Geometry: final body of the model. Coordinates: model frame, mm. Face numbers are marked on the shaded views. A direction names the side the tool comes from. Coordinates: 2 decimals unless noted, no trailing zeros. Loops run counter-clockwise (first coordinate to the right, second up) from the corner with the lowest first, then second, coordinate; pieces in that order, holes last. Notation, with made-up numbers: (27.25, -29.75) - (62.25, -29.75) arc R17 cw to (62.25, -9.75) - close; hole circle Ø8 at (42, -14.75). An arc over 180 degrees is marked (long way). Answer in a Markdown table with one row per item.
from build123d import *

# Parameters (mm, degrees)
F0_R     = 60
F1_DEPTH = 30


with BuildPart() as f1:
    # F0 (on Front) → F1 (new body)
    with BuildSketch(Plane.XZ):
        with BuildLine():
            Line((-23.376703, 94.018714), (-93.376703, 94.018714))
            Line((-93.376703, 94.018714), (-93.376703, 44.018714))
            ThreePointArc((-93.376703, 44.018714), (-119.373909, 14.018714), (-93.376703, -15.981286))
            Line((-93.376703, -15.981286), (-93.376703, -65.981286))
            Line((-93.376703, -65.981286), (-23.376703, -65.981286))
            Line((-23.376703, -65.981286), (-14.60776, -65.981286))
            ThreePointArc((-14.60776, -65.981286), (26.623297, -75.981286), (67.854353, -65.981286))
            Line((67.854353, -65.981286), (76.623297, -65.981286))
            Line((76.623297, -65.981286), (146.623297, -65.981286))
            Line((146.623297, -65.981286), (146.623297, -15.981286))
            ThreePointArc((146.623297, -15.981286), (166.623297, 14.018714), (146.623297, 44.018714))
            Line((146.623297, 44.018714), (146.623297, 94.018714))
            Line((146.623297, 94.018714), (76.623297, 94.018714))
            Line((76.623297, 94.018714), (67.854353, 94.018714))
            ThreePointArc((67.854353, 94.018714), (26.623297, 104.018714), (-14.60776, 94.018714))
            Line((-14.60776, 94.018714), (-23.376703, 94.018714))
        make_face()
        with BuildLine():
            ThreePointArc((-78.376703, 68.858823), (-75.447771, 75.92989), (-68.376703, 78.858823))
            Line((-68.376703, 78.858823), (-58.376703, 78.858823))
            ThreePointArc((-58.376703, 78.858823), (-51.305635, 75.92989), (-48.376703, 68.858823))
            Line((-48.376703, 68.858823), (-48.376703, -40.861128))
            ThreePointArc((-48.376703, -40.861128), (-51.305635, -47.932195), (-58.376703, -50.861128))
            Line((-58.376703, -50.861128), (-68.376703, -50.861128))
            ThreePointArc((-68.376703, -50.861128), (-75.447771, -47.932195), (-78.376703, -40.861128))
            Line((-78.376703, -40.861128), (-78.376703, 68.858823))
        make_face(mode=Mode.SUBTRACT)
        with BuildLine():
            ThreePointArc((101.623297, 68.858823), (104.552229, 75.92989), (111.623297, 78.858823))
            Line((111.623297, 78.858823), (121.623297, 78.858823))
            ThreePointArc((121.623297, 78.858823), (128.694365, 75.92989), (131.623297, 68.858823))
            Line((131.623297, 68.858823), (131.623297, -40.861128))
            ThreePointArc((131.623297, -40.861128), (128.694365, -47.932195), (121.623297, -50.861128))
            Line((121.623297, -50.861128), (111.623297, -50.861128))
            ThreePointArc((111.623297, -50.861128), (104.552229, -47.932195), (101.623297, -40.861128))
            Line((101.623297, -40.861128), (101.623297, 68.858823))
        make_face(mode=Mode.SUBTRACT)
        with Locations((26.623297, 14.018714)):
            Circle(F0_R, mode=Mode.SUBTRACT)
    extrude(amount=F1_DEPTH)


solid = f1.part
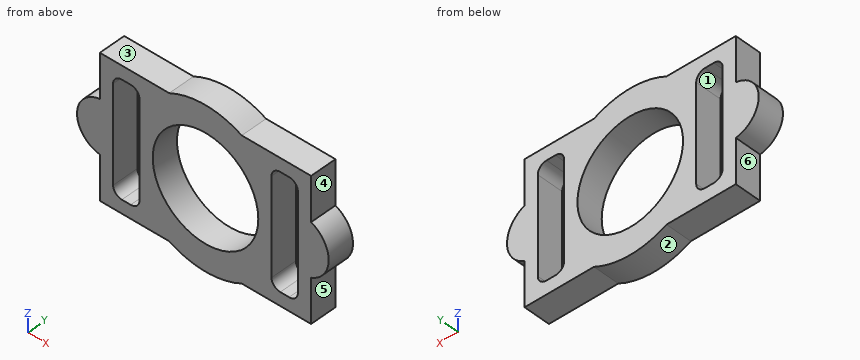
(1) Ray query, probe 1 along X at (y, z) = (-18.25, 52.5); probe 2 along X at (y, z) = (-8, 53); probe 3 along Z at (x, y) = (26, -25.75). Return the intervals inside material, ascending.
Verdict:
| item | result |
|---|---|
| probe 1 | x = -93.38 to -78.38, -48.38 to -19.41, 72.66 to 101.62, 131.62 to 146.62 |
| probe 2 | x = -93.38 to -78.38, -48.38 to -18.99, 72.24 to 101.62, 131.62 to 146.62 |
| probe 3 | z = -75.98 to -45.98, 74.02 to 104.02 |
(2) Access query for the marked faces 4, 5 and 6. Directions: +Z, -Z, +X, -X, +Y, -Y. A direction counts if a zero-diameter tool reaches every point of the face in a straight line with its end or side. Return the directions, or none.
Verdict:
| item | result |
|---|---|
| face 4 | +Z, +X, +Y, -Y |
| face 5 | -Z, +X, +Y, -Y |
| face 6 | -Z, -X, +Y, -Y |
(3) Pull-direction query (Z, two-part tool) for the marked faces 1, 2 and 3; classes: pulls with the +Z half, pulls with the -Z half, needs draft (parallel to the pull), parting line crosses it, or undercut.
Verdict:
| item | result |
|---|---|
| face 1 | undercut |
| face 2 | pulls with the -Z half |
| face 3 | pulls with the +Z half |
(4) Cut plane B-B on z = 20. Output: boundary loops of the cut face in (x, y).
Verdict:
| item | result |
|---|---|
| outline | (-118.78, -30) - (-78.38, -30) - (-78.38, 0) - (-118.78, 0) - close; (-48.38, -30) - (-33.08, -30) - (-33.08, 0) - (-48.38, 0) - close; (86.32, -30) - (101.62, -30) - (101.62, 0) - (86.32, 0) - close; (131.62, -30) - (166.07, -30) - (166.07, 0) - (131.62, 0) - close |
(5) Cut plane D-D on x = -22. Output: boundary loops of the cut face in (y, z), then the cut area to 3 significant figures.
Verdict:
| item | result |
|---|---|
| outline | (-30, -65.98) - (0, -65.98) - (0, -21.13) - (-30, -21.13) - close; (-30, 49.17) - (0, 49.17) - (0, 94.02) - (-30, 94.02) - close |
| area | 2,690 mm² |
(6) Cut plane A-A on x = 118.5. Output: boundary loops of the cut face in (y, z), then the cut area to 3 significant figures.
Verdict:
| item | result |
|---|---|
| outline | (-30, -65.98) - (0, -65.98) - (0, -50.86) - (-30, -50.86) - close; (-30, 78.86) - (0, 78.86) - (0, 94.02) - (-30, 94.02) - close |
| area | 908 mm² |
(7) First-contact query: pin 1 Ø3 at (y, z) = (-13, -40.5) entering from +X; pin 2 Ø8 at (x, z) = (6, 68) entering from -Y; pin 3 Ø3 at (x, y) = (42, -11) entering from -Z; pin 4 Ø11 at (x, y) = (117, -10) entering from +Z. Flat tips, straight axial feed; report the tip coordinate or a pass-through.
Verdict:
| item | result |
|---|---|
| pin 1 | stops at x = 146.62 |
| pin 2 | stops at y = -30 |
| pin 3 | stops at z = -74.91 |
| pin 4 | stops at z = 94.02 |
(8) Cut plane C-C on y = -7. State how many separate pieces and enclosed holes the cut face has, then the cut area to 3 significant figures.
Verdict:
| item | result |
|---|---|
| separate pieces | 1 |
| enclosed holes | 3 |
| area | 22,600 mm² |
